```python
from build123d import *

# Parameters (mm, degrees)
SKETCH1_W           = 65.9892
SKETCH1_H           = 4.4958
BOSS_EXTRUDE1_DEPTH = 20.4978
SKETCH4_W           = 65.9892
SKETCH4_H           = 2.0066
BOSS_EXTRUDE2_DEPTH = 4.8006
SKETCH5_R           = 1.11252
BOSS_EXTRUDE3_DEPTH = 37.8968


with BuildPart() as part:
    # Sketch1 → Boss-Extrude1 (new body)
    with BuildSketch(Plane.XY):
        Rectangle(SKETCH1_W, SKETCH1_H)
    extrude(amount=BOSS_EXTRUDE1_DEPTH)

    # Sketch4 → Boss-Extrude2 (add)
    with BuildSketch(Plane.XY.offset(20.4978)):
        with Locations((0, -1.2446)):
            Rectangle(SKETCH4_W, SKETCH4_H)
    extrude(amount=BOSS_EXTRUDE2_DEPTH)

    # Sketch5 → Boss-Extrude3 (add, symmetric)
    with BuildSketch(Plane(origin=(0, 0, 0), x_dir=(0, 0, -1), z_dir=(1, 0, 0))):
        with Locations((-2.4892, 0.3429)):
            Circle(SKETCH5_R)
    extrude(amount=BOSS_EXTRUDE3_DEPTH, both=True)


solid = part.part
```
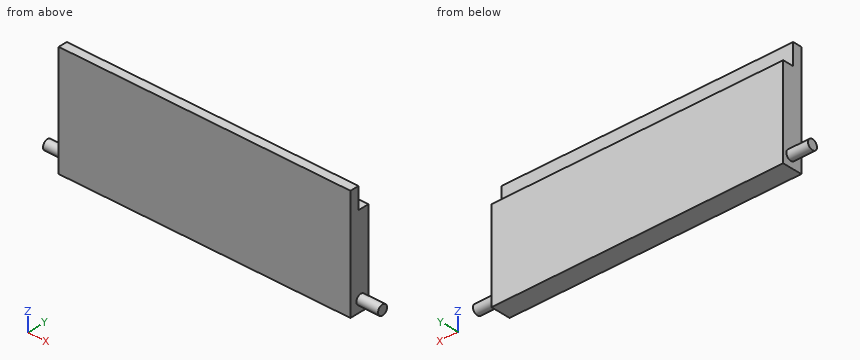
Verification items for the finished model (mm, model axes). Round coordinates to 2 decimals unless told otherwise and drop trailing zeros. Write each loop counter-clockwise with the first axis right and the second up, starting at its lowest first coordinate (ties: lowest second). Pieces come first, ordered by that corner, then holes.
1. Section check C-C on y = -1.6. Enter the section's corners in (x, z).
2. Gauge pin test, flat ends, axial feed: P1, Ø1.5, axis at y = -0.5, z = 5, coming from the -X side; P2, Ø1.4, axis at x = 4, z = 22, coming from the +Y side. Record the tip position at first contact, or that the pin passes through.
3. Section check B-B on z = 4.75. Enter the section's corners in (x, y).
4. Section check A-A on x = 4. Enter the section's corners in (y, z), plus the area to 3 significant figures.
5. Scan lines: L1, parallel to Z at x = -11.5, y = 0.7; L2, parallel to Y at x = -22, z = 21.5; L3, parallel to X at y = 0.1, z = 18. Record each from-to range of solid material in increasing order.
Answer:
1. outline: (-32.99, 0) - (32.99, 0) - (32.99, 25.3) - (-32.99, 25.3) - close
2. P1: stops at x = -32.99
2. P2: stops at y = -0.24
3. outline: (-32.99, -2.25) - (32.99, -2.25) - (32.99, 2.25) - (-32.99, 2.25) - close
4. outline: (-2.25, 0) - (2.25, 0) - (2.25, 20.5) - (-0.24, 20.5) - (-0.24, 25.3) - (-2.25, 25.3) - close
4. area: 102 mm2
5. L1: z = 0 to 20.5
5. L2: y = -2.25 to -0.24
5. L3: x = -32.99 to 32.99
